Design review of the part built by this model. Coordinates are the model's own, in mm. Face numbers are marked on the shaded views. A direction names the side the tool comes from. Coordinates: 2 decimals unless noted, no trailing zeros. Loops run counter-clockwise (first coordinate to the right, second up) from the corner with the lowest first, then second, coordinate; pieces in that order, holes last. Notation, with made-up numbers: M 0.5,40 L 40.5,40 A24 ccw 40.5,62 Z; hole C 86.5,14.25 d6. An arc over 180 degrees is marked long. Put each result on its own line as item: value. Start each with the question number.
(1) Take a section at B-B, the plane x = 0. Give the boundary of the cut face in (y, z).
(2) Take a section at C-C, the plane z = 1.5. Give the boundary of the cut face in (x, y), then the cut area to 3 significant figures.
(3) For the marked faces 1 and 2, list the 3-axis set-ups (+Z, -Z, +X, -X, +Y, -Y) from which the entire face can be reached by the end or side of a thin tool; tool diameter is ignored.
(4) Take a section at D-D, the plane z = 6.5. Give the boundary of the cut face in (x, y), then the cut area to 3 significant figures.
(5) Clearance check with flat-ended pins moving along their axes: pin 1 (6 mm diameter, centred on x = -12, y = -12, fed in from +Z); pin 2 (12 mm diameter, centred on x = -1, y = 45.5, fed in from +Z); pin 3 (3 mm diameter, centred on x = -20.5, z = 6.5, fed in from -Y). State where each tip first meets the part, or that it passes through.
(6) For probe 1 along Z at (x, y) = (-3, -4.5); probe 2 along Y at (x, z) = (20.5, 8.5); probe 3 along Y at (x, z) = (19, 7), list the stretches that pass through material, from the lowest coordinate up. Write a range as [from, to].
(7) The part is to be moulded in two halves that separate along Y. For the marked faces 3, 4 and 5, say which applies: +Y half, -Y half, draft (parallel to the pull), parting line (faces both ways), or undercut.
(8) Take a section at A-A, the plane y = 13. Give the boundary of the cut face in (x, z).
```python
from build123d import *

# Parameters (mm, degrees)
F1_DEPTH = 11.5
F2_R     = 8
F4_DEPTH = 0.5
F5_W     = 53
F5_H     = 88
F6_DEPTH = 0.1
F8_DEPTH = 0.2


with BuildPart() as f1:
    # F0 (on Top) → F1 (new body)
    with BuildSketch(Plane.XY):
        with BuildLine():
            ThreePointArc((32.75, 41), (26.892136, 55.142136), (12.75, 61))
            Line((12.75, 61), (-12.75, 61))
            ThreePointArc((-12.75, 61), (-26.892136, 55.142136), (-32.75, 41))
            Line((-32.75, 41), (-32.75, -41))
            ThreePointArc((-32.75, -41), (-26.892136, -55.142136), (-12.75, -61))
            Line((-12.75, -61), (12.75, -61))
            ThreePointArc((12.75, -61), (26.892136, -55.142136), (32.75, -41))
            Line((32.75, -41), (32.75, 41))
        make_face()
    extrude(amount=F1_DEPTH)

    # F2
    f2_edges = [f1.edges().sort_by_distance(p)[0] for p in [
        (-26.892136, 55.142136, 0),
    ]]
    fillet(f2_edges, radius=F2_R)

    # F3 (on face) → F4 (join)
    with BuildSketch(Plane.XY.offset(11.5)):
        with BuildLine():
            Line((0, -47), (-6.607793, -47))
            ThreePointArc((-6.607793, -47), (-7.419988, -47.416614), (-7.55544, -48.31932))
            Line((-7.55544, -48.31932), (-6.544556, -51.31932))
            ThreePointArc((-6.544556, -51.31932), (-6.180295, -51.812195), (-5.596909, -52))
            Line((-5.596909, -52), (0, -52))
            Line((0, -52), (5.596909, -52))
            ThreePointArc((5.596909, -52), (6.180295, -51.812195), (6.544556, -51.31932))
            Line((6.544556, -51.31932), (7.55544, -48.31932))
            ThreePointArc((7.55544, -48.31932), (7.419988, -47.416614), (6.607793, -47))
            Line((6.607793, -47), (0, -47))
        make_face()
    extrude(amount=F4_DEPTH)

    # F5 (on face) → F6 (join)
    with BuildSketch(Plane.XY.offset(11.5)):
        Rectangle(F5_W, F5_H)
    extrude(amount=F6_DEPTH)

    # F7 (on face) → F8 (join)
    with BuildSketch(Plane.XY.offset(11.5)):
        with BuildLine():
            Line((-5.75, 51.25), (5.75, 51.25))
            ThreePointArc((5.75, 51.25), (6.28033, 51.46967), (6.5, 52))
            ThreePointArc((6.5, 52), (6.28033, 52.53033), (5.75, 52.75))
            Line((5.75, 52.75), (-5.75, 52.75))
            ThreePointArc((-5.75, 52.75), (-6.28033, 52.53033), (-6.5, 52))
            ThreePointArc((-6.5, 52), (-6.28033, 51.46967), (-5.75, 51.25))
        make_face()
    extrude(amount=F8_DEPTH)


solid = f1.part
```
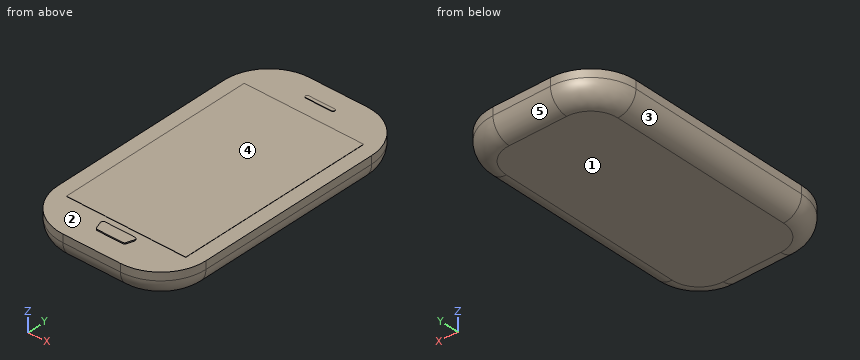
Computed values:
1. outline: M -61,8 A8 ccw -53,0 L 53,0 A8 ccw 61,8 L 61,11.5 L 52.75,11.5 L 52.75,11.7 L 51.25,11.7 L 51.25,11.5 L 44,11.5 L 44,11.6 L -44,11.6 L -44,11.5 L -47,11.5 L -47,12 L -52,12 L -52,11.5 L -61,11.5 Z
2. outline: M -29.41,-41 A16.66 ccw -12.75,-57.66 L 12.75,-57.66 A16.66 ccw 29.41,-41 L 29.41,41 A16.66 ccw 12.75,57.66 L -12.75,57.66 A16.66 ccw -29.41,41 Z
2. area: 6,550 mm^2
3. face 1: -Z, +X, -X, +Y, -Y
3. face 2: +Z
4. outline: M -32.61,-41 A19.86 ccw -12.75,-60.86 L 12.75,-60.86 A19.86 ccw 32.61,-41 L 32.61,41 A19.86 ccw 12.75,60.86 L -12.75,60.86 A19.86 ccw -32.61,41 Z
4. area: 7,600 mm^2
5. pin 1: stops at z = 11.6
5. pin 2: stops at z = 11.7
5. pin 3: stops at y = -59.9
6. probe 1: z = [0, 11.6]
6. probe 2: y = [-59.44, 59.44]
6. probe 3: y = [-59.93, 59.93]
7. face 3: draft
7. face 4: undercut
7. face 5: +Y half
8. outline: M -32.75,8 A8 ccw -24.75,0 L 24.75,0 A8 ccw 32.75,8 L 32.75,11.5 L 26.5,11.5 L 26.5,11.6 L -26.5,11.6 L -26.5,11.5 L -32.75,11.5 Z
